Solid Edge part; units mm, degrees
sketch "Sketch1" plane through (0, 0, 0) normal (1, 0, 0) x (0, 1, 0)
  line L0 (0, 50) -> (0, 34)
  line L1 (0, 34) -> (-5, 34)
  line L2 (-5, 34) -> (-5, 0)
  line L3 (-5, 0) -> (4, 0)
  line L4 (8, 0) -> (4, 0)
  line L5 (8, 34) -> (8, 0)
  line L6 (8, 34) -> (8, 50)
  line L7 (0, 50) -> (8, 50)
revolve "RevolvedProtrusion1" add sketch "Sketch1" angle 360 about axis through (0, -22.1591, 0) along (0, 1, 0)
revolve "RevolvedProtrusion2" [suppressed]
hole "Hole1" at (29.6985, 8, -29.6985) direction (0, -1, 0) diameter 8.5 end through all
hole "Hole2" at (-29.6985, 8, -29.6985) direction (0, -1, 0) diameter 8.5 end through all
hole "Hole3" at (29.6985, 8, 29.6985) direction (0, -1, 0) diameter 8.5 end through all
hole "Hole4" at (-29.6985, 8, 29.6985) direction (0, -1, 0) diameter 8.5 end through all
Geometry check sheet. Reference: the model listing, model coordinates, mm. A direction names the side the tool comes from. Round coordinates to 2 decimals unless told otherwise and drop trailing zeros. Order: outer loops, then holes, each group sorted by start corner. A loop starts at its lowest first (then second) coordinate and runs counter-clockwise, first axis right, second up. Notation, with made-up numbers: (74, -22) - (121, -22) arc R28 ccw to (121, 11) - close; hole circle Ø8 at (-5, 9.25). An arc over 180 degrees is marked (long way). One line per question, with ' | ' between items. Start each with the question number.
(1) Sectioned sample at C-C on x = 0. Record the cut outline in (y, z).
(2) Access from +Z, -Z, +X, -X, +Y, -Y to the whole of each face (thin tool, end or side, straight path). Record for faces 1 (the flat face through (0, -5, 0)), 2 (the flat face through (-33, 0, 10)).
(3) Sectioned sample at D-D on y = 5. Record the cut outline in (x, z).
(4) Thickness scan on L1, parallel to X at y = 2, z = 26; L2, parallel to X at y = 5.75, z = 32. Record the ranges inside material, lowest first. Write a range as [from, to].
(5) Depth check by flat-ended pin: pin 1 Ø13.5 at (x, z) = (-29.7, 29.7) entering from -Y; pin 2 Ø5 at (x, z) = (-29.7, -29.7) entering from -Y (3 decimals); pin 3 Ø3 at (y, z) = (6, -40) entering from -X; pin 4 Ø1 at (y, z) = (5, 2.5) entering from +X. Enter the tip coordinate at first touch or a pass-through.
(6) Release check for a two-part mould opening along X. For faces 3 (the flat face through (1, 8, -1)), 4 (the cylindrical face through (-33.847, 4.056, -30.62)), 5 (the cylindrical face through (-28.67, -2.54, 18.28)) record: released by +X, released by -X, zero draft, split by the parting line, or undercut.
(7) Sectioned sample at B-B on z = 0. Record the cut outline in (x, y).
(8) Sectioned sample at A-A on x = 27. Record the cut outline in (y, z).
Conclusion:
1) outline: (-5, -34) - (0, -34) - (0, -50) - (8, -50) - (8, 50) - (0, 50) - (0, 34) - (-5, 34) - close
2) face 1: +Z, -Z, +X, -X, -Y | face 2: -Y
3) outline: circle Ø100 at (0, 0); hole circle Ø8.5 at (-29.7, -29.7); hole circle Ø8.5 at (-29.7, 29.7); hole circle Ø8.5 at (29.7, -29.7); hole circle Ø8.5 at (29.7, 29.7)
4) L1: x = [-42.71, -31.79], [-27.6, 27.6], [31.79, 42.71] | L2: x = [-38.42, -33.27], [-26.13, 26.13], [33.27, 38.42]
5) pin 1: stops at y = 0 | pin 2: passes through | pin 3: stops at x = -31.9 | pin 4: stops at x = 49.96
6) face 3: zero draft | face 4: undercut | face 5: split by the parting line
7) outline: (-50, 0) - (-34, 0) - (-34, -5) - (34, -5) - (34, 0) - (50, 0) - (50, 8) - (-50, 8) - close
8) outline: (-5, -20.66) - (0, -20.66) - (0, -26.42) - (8, -26.42) - (8, 26.42) - (0, 26.42) - (0, 20.66) - (-5, 20.66) - close; (0, -42.08) - (8, -42.08) - (8, -32.98) - (0, -32.98) - close; (0, 32.98) - (8, 32.98) - (8, 42.08) - (0, 42.08) - close
